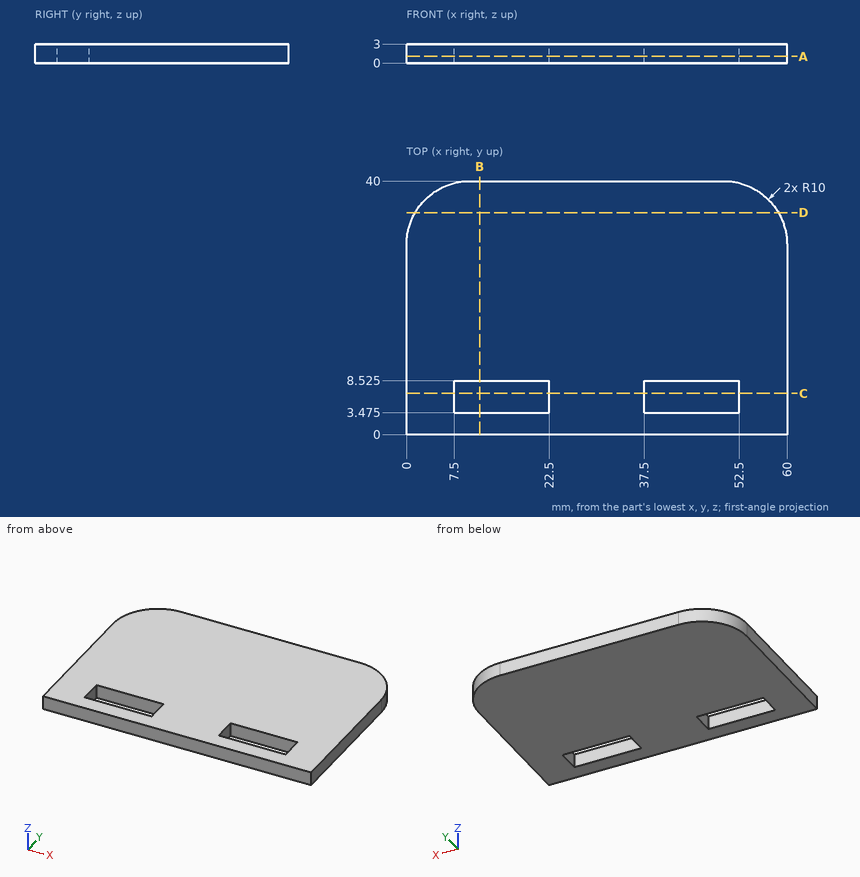
Source: three-view drawing plus pictorial views. Frame: mm from the lowest corner of the part. Coordinates: 2 decimals unless noted, no trailing zeros. Loops run counter-clockwise (first coordinate to the right, second up) from the corner with the lowest first, then second, coordinate; pieces in that order, holes last. Notation, with made-up numbers: (61, -35.5) - (76, -35.5) arc R26 ccw to (76, -7.5) - close; hole circle Ø11 at (-14, -30). An arc over 180 degrees is marked (long way). One line per item, written item: value. Start each with the question number.
1. Section A-A (z = 1.05). Return the cut outline in (x, y) (3 decimals).
2. Contact query for a flat-ended pin moving along its axis: P1, Ø1.5, axis at x = 46, z = 1.5, coming from the -Y side. Output: stop coordinate, or through.
3. Section B-B (x = 11.5). Return the cut outline in (y, z) (3 decimals), and give its area (3 significant figures).
4. Section D-D (y = 35). Return the cut outline in (x, z).
5. Section C-C (y = 6.5). Return the cut outline in (x, z).
6. Ray query, L1, parallel to Y at x = 17, z = 1 (3 decimals); L2, parallel to Y at x = 8, z = 0.6 (3 decimals); L3, parallel to X at y = 38.5, z = 2.7. Return the intervals inside material, ascending.
Verdict:
1. outline: (0, 0) - (60, 0) - (60, 30) arc R10 ccw to (50, 40) - (10, 40) arc R10 ccw to (0, 30) - close; hole (7.5, 3.475) - (22.5, 3.475) - (22.5, 8.525) - (7.5, 8.525) - close; hole (37.5, 3.475) - (52.5, 3.475) - (52.5, 8.525) - (37.5, 8.525) - close
2. P1: stops at y = 0
3. outline: (0, 0) - (3.475, 0) - (3.475, 3) - (0, 3) - close; (8.525, 0) - (40, 0) - (40, 3) - (8.525, 3) - close
3. area: 105 mm2
4. outline: (1.34, 0) - (58.66, 0) - (58.66, 3) - (1.34, 3) - close
5. outline: (0, 0) - (7.5, 0) - (7.5, 3) - (0, 3) - close; (22.5, 0) - (37.5, 0) - (37.5, 3) - (22.5, 3) - close; (52.5, 0) - (60, 0) - (60, 3) - (52.5, 3) - close
6. L1: y = 0 to 3.475, 8.525 to 40
6. L2: y = 0 to 3.475, 8.525 to 39.798
6. L3: x = 4.73 to 55.27
